Input: part model. Units: mm. Frame: model coordinates. Face numbers are marked on the shaded views. A direction names the side the tool comes from. Round coordinates to 2 decimals unless told otherwise and drop trailing zeros. Write each loop counter-clockwise with the first axis right and the second up, starting at its lowest first coordinate (ties: lowest second). Pieces come first, ordered by that corner, then holes. Notation, with made-up numbers: (22.25, 56) - (30.25, 56) arc R18 cw to (30.25, 86) - close; hole circle Ø6 at (1, 32.5). An arc over 180 degrees is marked (long way). Use one line per item in the form item = value.
```python
from build123d import *

# Parameters (mm, degrees)
F0_W     = 28
F0_H     = 6
F0_R     = 1.75
F1_DEPTH = 2
F2_W     = 2
F2_H     = 6
F3_DEPTH = 5
F4_SIZE  = 1
F5_R     = 2


with BuildPart() as f1:
    # F0 (on Top) → F1 (new body)
    with BuildSketch(Plane.XY):
        Rectangle(F0_W, F0_H)
        with Locations((10, 0)):
            Circle(F0_R, mode=Mode.SUBTRACT)
    extrude(amount=F1_DEPTH)

    # F2 (on face) → F3 (join)
    with BuildSketch(Plane(origin=(0, 0, 0), x_dir=(1, 0, 0), z_dir=(0, 0, -1))):
        with Locations((-1, 0)):
            Rectangle(F2_W, F2_H)
    extrude(amount=F3_DEPTH)

    # F4
    f4_edges = [f1.edges().sort_by_distance(p)[0] for p in [
        (8.25, 0, 2),
    ]]
    chamfer(f4_edges, length=F4_SIZE)

    # F5
    f5_edges = [f1.edges().sort_by_distance(p)[0] for p in [
        (14, -3, 1),
        (-14, -3, 1),
        (-14, 3, 1),
        (14, 3, 1),
    ]]
    fillet(f5_edges, radius=F5_R)


solid = f1.part
```
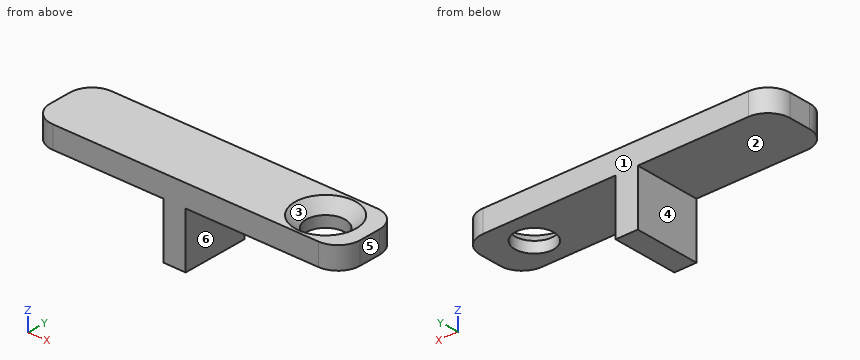
(1) First-contact query: pin 1 Ø1 at (x, y) = (-4, -1) entering from -Z; pin 2 Ø1.5 at (y, z) = (-1, -2.5) entering from +X; pin 3 Ø1.5 at (y, z) = (1.5, -3.5) entering from -X. Flat tips, straight axial feed; report the tip coordinate or a pass-through.
Derived:
pin_1 = 0
pin_2 = 0
pin_3 = -2
(2) Access query for the marked faces 4, 5 and 6. Directions: +Z, -Z, +X, -X, +Y, -Y. A direction counts if a zero-diameter tool reaches every point of the face in a straight line with its end or side. Return the directions, or none.
Derived:
face_4 = -Z, -X, +Y, -Y
face_5 = +Z, -Z, +X, +Y, -Y
face_6 = -Z, +X, +Y, -Y
(3) Cut plane C-C on z = -1.5. Output: boundary loops of the cut face in (x, y), then the cut area to 3 significant figures.
Derived:
outline = (-2, -3) - (0, -3) - (0, 3) - (-2, 3) - close
area = 12.0 mm^2
(4) Cut plane D-D on x = -2.5. Output: boundary loops of the cut face in (y, z).
Derived:
outline = (-3, 0) - (3, 0) - (3, 2) - (-3, 2) - close
(5) Cut plane A-A on y = 0. Output: boundary loops of the cut face in (x, z), then the cut area to 3 significant figures.
Derived:
outline = (-14, 0) - (-2, 0) - (-2, -5) - (0, -5) - (0, 0) - (8.25, 0) - (8.25, 1) - (7.25, 2) - (-14, 2) - close; (11.75, 0) - (14, 0) - (14, 2) - (12.75, 2) - (11.75, 1) - close
area = 58.0 mm^2
(6) Draft query along Y for the marked faces 1, 2 and 3. Return one class per face: released by +Y, released by -Y, zero draft, split by the parting line, or undercut.
Derived:
face_1 = released by +Y
face_2 = zero draft
face_3 = undercut
(7) Cut plane B-B on x = 10. Output: boundary loops of the cut face in (y, z).
Derived:
outline = (-3, 0) - (-1.75, 0) - (-1.75, 1) - (-2.75, 2) - (-3, 2) - close; (1.75, 0) - (3, 0) - (3, 2) - (2.75, 2) - (1.75, 1) - close
(8) Material intervals for L1, parallel to Y at x = 10, z = 0.4; L2, parallel to Z at x = 2, y = -1; L3, parallel to X at y = 1, z = -0.25, sorted ascending.
Derived:
L1 = -3 to -1.75, 1.75 to 3
L2 = 0 to 2
L3 = -2 to 0
